from build123d import *

# Parameters (mm, degrees)
SKETCH_1_W                = 178
SKETCH_1_H                = 25
SKETCH_6_OUTSIDE_W        = 90.306
SKETCH_6_OUTSIDE_H        = 90.306
SKETCH_6_OUTSIDE_W_2      = 44
SKETCH_6_OUTSIDE_H_2      = 60
CUT_EXTRUDE_1_DEPTH       = 20
M26X1_5_2_D               = 23.5
SKETCH_10_R               = 45
SKETCH_10_R_2             = 25
EXTRUDE_1_DEPTH           = 10
HOLE_WIZARD_1_D           = 6.6
HOLE_WIZARD_1_CBORE_D     = 11
HOLE_WIZARD_1_CBORE_DEPTH = 6.8
PATTERN_CIRCULAR_1_COUNT  = 4
SKETCH_14_R               = 17.5
CUT_EXTRUDE_2_DEPTH       = 120


with BuildPart() as part:
    # 草图1 → 旋转1 (revolve)
    with BuildSketch(Plane.XY):
        with Locations((89, 12.5)):
            Rectangle(SKETCH_1_W, SKETCH_1_H)
    revolve(axis=Axis((-8.837336018, 0, 0), (1, 0, 0)))

    # 草图6 outside → 切除-拉伸1 (cut)
    with BuildSketch(Plane.ZY):
        Rectangle(SKETCH_6_OUTSIDE_W, SKETCH_6_OUTSIDE_H)
        Rectangle(SKETCH_6_OUTSIDE_W_2, SKETCH_6_OUTSIDE_H_2, mode=Mode.SUBTRACT)
    extrude(amount=-CUT_EXTRUDE_1_DEPTH, mode=Mode.SUBTRACT)

    # M26x1.5螺纹孔2 (through all)
    with Locations(Plane.ZY):
        with Locations((0, 0)):
            Hole(M26X1_5_2_D / 2)

    # 草图10 → 凸台-拉伸1 (add)
    with BuildSketch(Plane(origin=(178, 0, 0), x_dir=(0, 0, -1), z_dir=(1, 0, 0))):
        Circle(SKETCH_10_R)
        Circle(SKETCH_10_R_2, mode=Mode.SUBTRACT)
    extrude(amount=-EXTRUDE_1_DEPTH)

    # 打孔尺寸(%根据)内六角圆柱头螺钉的类型1 (through all)
    with Locations(Plane(origin=(168, 35, 0), x_dir=(0, 0, -1), z_dir=(-1, 0, 0))):
        with Locations((0, 0)):
            hole_wizard_1 = CounterBoreHole(HOLE_WIZARD_1_D / 2, HOLE_WIZARD_1_CBORE_D / 2, HOLE_WIZARD_1_CBORE_DEPTH)

    # 阵列(圆周)1: 打孔尺寸(%根据)内六角圆柱头螺钉的类型1 ×4 about axis
    pattern_circular_1_axis = Axis((0, 0, 0), (1, 0, 0))
    for i in range(1, PATTERN_CIRCULAR_1_COUNT):
        add(hole_wizard_1.rotate(pattern_circular_1_axis, i * 360 / PATTERN_CIRCULAR_1_COUNT), mode=Mode.SUBTRACT)

    # 草图14 → 切除-拉伸2 (cut)
    with BuildSketch(Plane(origin=(178, 0, 0), x_dir=(0, 0, -1), z_dir=(1, 0, 0))):
        Circle(SKETCH_14_R)
    extrude(amount=-CUT_EXTRUDE_2_DEPTH, mode=Mode.SUBTRACT)


solid = part.part
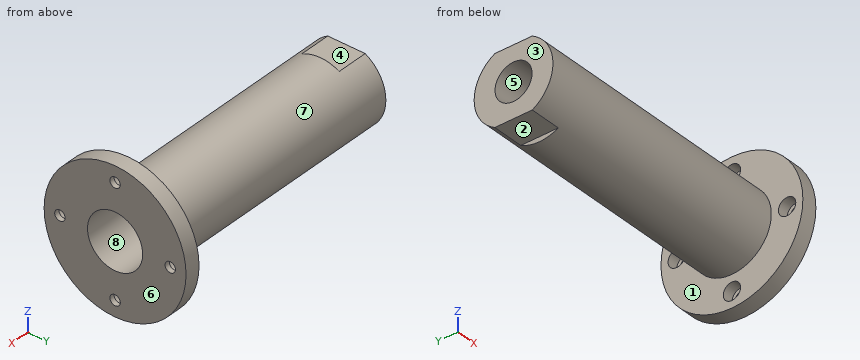
For this review, take the finished solid that the model builds, in its own axes (mm). Face numbers are marked on the shaded views. A direction names the side the tool comes from. Coordinates: 2 decimals unless noted, no trailing zeros. Loops run counter-clockwise (first coordinate to the right, second up) from the corner with the lowest first, then second, coordinate; pieces in that order, holes last. Notation, with made-up numbers: (-2.75, -5) - (35.25, -5) arc R11 cw to (35.25, 7) - close; hole circle Ø11 at (-11.75, 68). An arc over 180 degrees is marked (long way). Use a Markdown table: item, result. Add a question column.
Item 1: We need section D-D (y = 15). Give the boundary of the cut face in (x, z), and give its area (3 significant figures).
Item 2: We need section C-C (z = 35). Give the boundary of the cut face in (x, y), and give its area (3 significant figures).
Item 3: For line 1 (Y direction, x = 177, z = 0); line 2 (Y direction, x = 140, z = -1); line 3 (X direction, y = 8.5, z = 14), list the stretches that pass through material, from the lowest coordinate up.
Item 4: Insertion check: pin 1 Ø2.5 at (y, z) = (5.5, 23.5) entering from -X; pin 2 Ø12 at (y, z) = (0, -34.5) entering from -X; pin 3 Ø10 at (x, z) = (106, 22.5) entering from +Y; pin 4 Ø12 at (y, z) = (3, -12.5) entering from -X. Each pin has a flat end and moves straight along its axis. Give the tip position at first contact, or say it passes through.
Item 5: Tool access review of the marked faces 1, 2, 3 and 4: name each direction out of +Z, -Z, +X, -X, +Y, -Y from which nothing blocks a thin tool from reaching the whole face with its end or side.
Item 6: We need section A-A (z = 0). Give the number of separate pieces and of enclosed holes in the cut face, and give its area (3 significant figures).
Item 7: Mouldability with a two-part tool opening along Y and no side actions: class the marked faces 5, 6, 7 and 8 as pulls with the +Y half, pulls with the -Y half, needs draft (parallel to the pull), parting line crosses it, or undercut.
Item 8: We need section B-B (x = 12.5). Give the boundary of the cut face in (y, z).
Results list:
| question | item | result |
|---|---|---|
| 1 | outline | (0, -20) - (168, -20) - (168, -42.43) - (178, -42.43) - (178, -9.01) - (58, -9.01) - (58, 9.01) - (178, 9.01) - (178, 42.43) - (168, 42.43) - (168, 20) - (0, 20) - close |
| 1 | area | 5,410 mm^2 |
| 2 | outline | (168, -28.28) - (178, -28.28) - (178, -3.3) - (174.8, -3.3) - (174.8, -5.5) - (168, -5.5) - close; (168, 5.5) - (174.8, 5.5) - (174.8, 3.3) - (178, 3.3) - (178, 28.28) - (168, 28.28) - close |
| 2 | area | 470 mm^2 |
| 3 | line 1 | y = -45 to -38.3, -31.7 to -17.5, 17.5 to 31.7, 38.3 to 45 |
| 3 | line 2 | y = -24.98 to -17.47, 17.47 to 24.98 |
| 3 | line 3 | x = 0 to 58 |
| 4 | pin 1 | stops at x = 20 |
| 4 | pin 2 | stops at x = 168 |
| 4 | pin 3 | stops at y = 17.85 |
| 4 | pin 4 | stops at x = 0 |
| 5 | face 1 | -X |
| 5 | face 2 | -Z, -X, +Y, -Y |
| 5 | face 3 | +Z, -Z, -X, +Y, -Y |
| 5 | face 4 | +Z, -X, +Y, -Y |
| 6 | separate pieces | 4 |
| 6 | enclosed holes | 0 |
| 6 | area | 3,550 mm^2 |
| 7 | face 5 | undercut |
| 7 | face 6 | needs draft |
| 7 | face 7 | parting line crosses it |
| 7 | face 8 | undercut |
| 8 | outline | (-11.87, -22) - (11.87, -22) arc R25 ccw to (11.87, 22) - (-11.87, 22) arc R25 ccw to start; hole circle Ø23.5 at (0, 0) |
